```python
from build123d import *

# Parameters (mm, degrees)
RESSALTO_EXTRUS_O2_DEPTH = 5
ESBO_O4_R                = 4.25
CORTE_EXTRUS_O1_DEPTH    = 4
ESBO_O5_R                = 1.5
CORTE_EXTRUS_O2_DEPTH    = 7
ESBO_O6_R                = 7.5
CORTE_EXTRUS_O3_DEPTH    = 11


with BuildPart() as part:
    # Esboço3 → Ressalto-extrusão2 (new body, symmetric)
    with BuildSketch(Plane.XY):
        with BuildLine():
            Line((0, 50), (98.5, 105))
            ThreePointArc((98.5, 105), (109.596194078, 109.596194078), (105, 98.5))
            Line((105, 98.5), (50, 0))
            Line((50, 0), (0, 0))
            Line((0, 0), (0, 50))
        make_face()
    extrude(amount=RESSALTO_EXTRUS_O2_DEPTH, both=True)

    # Esboço4 → Corte-extrusão1 (cut)
    with BuildSketch(Plane.XY.offset(5)):
        with Locations((105, 105)):
            Circle(ESBO_O4_R)
    extrude(amount=-CORTE_EXTRUS_O1_DEPTH, mode=Mode.SUBTRACT)

    # Esboço5 → Corte-extrusão2 (cut, through all)
    with BuildSketch(Plane.XY.offset(1)):
        with Locations((105, 105)):
            Circle(ESBO_O5_R)
    extrude(amount=-CORTE_EXTRUS_O2_DEPTH, mode=Mode.SUBTRACT)

    # Esboço6 → Corte-extrusão3 (cut, through all)
    with BuildSketch(Plane.XY.offset(5)):
        with Locations((14.825558834, 35.174441166)):
            Circle(ESBO_O6_R)
        with Locations((35.174441166, 14.825558834)):
            Circle(ESBO_O6_R)
    extrude(amount=-CORTE_EXTRUS_O3_DEPTH, mode=Mode.SUBTRACT)


with BuildPart() as body_2:
    # Espelhar1: mirrored copy
    add(part.part.mirror(Plane(origin=(0, 0, 5), x_dir=(0, 0, 1), z_dir=(0, 1, 0))))


with BuildPart() as body_3:
    # Espelhar2: mirrored copy
    add(body_2.part.mirror(Plane(origin=(0, 0, 5), x_dir=(0, 0, 1), z_dir=(1, 0, 0))))


with BuildPart() as body_4:
    # Espelhar2 2: mirrored copy
    add(part.part.mirror(Plane(origin=(0, 0, 5), x_dir=(0, 0, 1), z_dir=(1, 0, 0))))


solid = body_4.part
```
Work out the finished part from the listing and answer in its coordinate system (mm). A direction names the side the tool comes from. Round coordinates to 2 decimals unless told otherwise and drop trailing zeros. Order: outer loops, then holes, each group sorted by start corner. A loop starts at its lowest first (then second) coordinate and runs counter-clockwise, first axis right, second up.
Q1. Find the intervals of material crossed by line 1 along Y through (x, z) = (-105, -1.1); line 2 along X through (y, z) = (105, -2.8); line 3 along Y through (x, z) = (-105, 2.4), in increasing order.
Solution:
line 1: y = 98.5 to 103.5, 106.5 to 111.5
line 2: x = -111.5 to -106.5, -103.5 to -98.5
line 3: y = 98.5 to 100.75, 109.25 to 111.5
Q2. A cutting plane is placed at A-A, the plane y = 10.5. Determine the outline of the cut face in (x, z), then the cut area to 3 significant figures.
Solution:
outline: (-55.86, -5) - (-41.3, -5) - (-41.3, 5) - (-55.86, 5) - close; (-29.05, -5) - (0, -5) - (0, 5) - (-29.05, 5) - close
area: 436 mm2
Q3. A tool of negligible diameter and unlimited length cuts with its end or side. For faces 5 (the cylindrical face through (-100.754, 105.187, 3.028)), 6 (the flat face through (-48.561, 77.115, 0.07)), from which of +Z, -Z, +X, -X, +Y, -Y can it reach the whole face along a straight path? Write none if from no direction.
Solution:
face 5: +Z
face 6: +Z, -Z, +X, +Y
Q4. The mould has two halves that part along X. Classify faces 1 (the cylindrical face through (-104.805, 106.487, -1.958)), 2 (the cylindrical face through (-109.442, 109.745, 0.07)), 3 (the flat face through (-107, 105, 1)), 4 (the flat face through (-77.885, 49.939, 0.07)): pulls with the +X half, pulls with the -X half, needs draft (parallel to the pull), parting line crosses it, or undercut.
Solution:
face 1: undercut
face 2: parting line crosses it
face 3: undercut
face 4: pulls with the -X half
Q5. Given pin 1 Ø5 at (y, z) = (17, 2.5) entering from -X; pin 2 Ø6 at (x, z) = (-43, 1) entering from +Y; pin 3 Ø6 at (y, z) = (92, -3.5) entering from +X, each flat-ended and moving along its own axis, determine where each tip first touches the part or whether it passes through.
Solution:
pin 1: stops at x = -60.89
pin 2: stops at y = 75.69
pin 3: stops at x = -69.85
Q6. A cutting plane is placed at C-C, the plane x = -93. Determine the outline of the cut face in (y, z), then the cut area to 3 significant figures.
Solution:
outline: (77.01, -5) - (101.93, -5) - (101.93, 5) - (77.01, 5) - close
area: 249 mm2
Q7. A cutting plane is placed at B-B, the plane z = -2.75. Determine the outline of the cut face in (x, y), then the cut area to 3 significant figures.
Solution:
outline: (-105, 98.5) - (-50, 0) - (0, 0) - (0, 50) - (-98.5, 105) arc R6.5 ccw (long way) to start; hole circle Ø3 at (-105, 105); hole circle Ø15 at (-35.17, 14.83); hole circle Ø15 at (-14.83, 35.17)
area: 5,350 mm2
Q8. A cutting plane is placed at D-D, the plane y = 48.5. Determine the outline of the cut face in (x, z).
Solution:
outline: (-77.08, -5) - (0, -5) - (0, 5) - (-77.08, 5) - close
